Design review of the part built by this model. Coordinates are the model's own, in mm. Face numbers are marked on the shaded views. A direction names the side the tool comes from. Give positions to 0.01 mm unless a question says otherwise; leave off trailing zeros. Order: outer loops, then holes, each group sorted by start corner. A loop starts at its lowest first (then second) coordinate and runs counter-clockwise, first axis right, second up.
```python
from build123d import *

# Parameters (mm, degrees)
SKETCH1_R           = 14
BOSS_EXTRUDE1_DEPTH = 25
SKETCH3_R           = 4.5
BOSS_EXTRUDE2_DEPTH = 1
SKETCH4_R           = 1
CUT_EXTRUDE1_DEPTH  = 4
SKETCH5_R           = 1.5
CUT_EXTRUDE2_DEPTH  = 4


with BuildPart() as part:
    # Sketch1 → Boss-Extrude1 (new body)
    with BuildSketch(Plane(origin=(0, 0, 0), x_dir=(1, 0, 0), z_dir=(0, 1, 0))):
        with Locations(Location((0, 0, 0), (0, 0, 270))):
            Circle(SKETCH1_R)
    extrude(amount=BOSS_EXTRUDE1_DEPTH)

    # Sketch3 → Boss-Extrude2 (add)
    with BuildSketch(Plane(origin=(0, 25, 0), x_dir=(1, 0, 0), z_dir=(0, 1, 0))):
        with Locations(Location((0, 0, 0), (0, 0, 270))):
            Circle(SKETCH3_R)
    extrude(amount=BOSS_EXTRUDE2_DEPTH)

    # Sketch4 → Cut-Extrude1 (cut)
    with BuildSketch(Plane(origin=(0, 25, 0), x_dir=(1, 0, 0), z_dir=(0, 1, 0))):
        with Locations(Location((0, 5.773502692, 0), (0, 0, 270))):
            Circle(SKETCH4_R)
        with Locations(Location((5, -2.886751346, 0), (0, 0, 270))):
            Circle(SKETCH4_R)
        with Locations(Location((-5, -2.886751346, 0), (0, 0, 270))):
            Circle(SKETCH4_R)
    extrude(amount=-CUT_EXTRUDE1_DEPTH, mode=Mode.SUBTRACT)

    # Sketch5 → Cut-Extrude2 (cut)
    with BuildSketch(Plane.XZ):
        with Locations(Location((9.5, 0, 0), (0, 0, 270))):
            Circle(SKETCH5_R)
        with Locations(Location((-9.5, 0, 0), (0, 0, 270))):
            Circle(SKETCH5_R)
        with Locations(Location((0, -8, 0), (0, 0, 270))):
            Circle(SKETCH5_R)
        with Locations(Location((0, 8, 0), (0, 0, 270))):
            Circle(SKETCH5_R)
    extrude(amount=-CUT_EXTRUDE2_DEPTH, mode=Mode.SUBTRACT)


solid = part.part
```
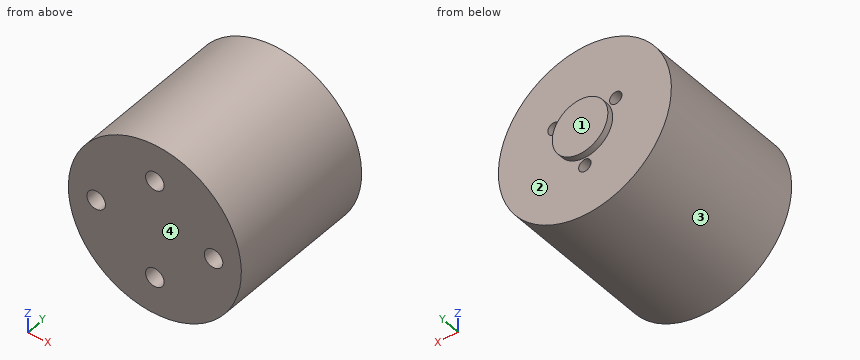
1. Take a section at D-D (y = 20). State the section outline as (x, z) points.
Recorded:
outline: circle Ø28 at (0, 0)
2. Draft analysis for pull direction Z (two halves, no side actions). For the marked faces 3 and 4, state which applies: pulls with the +Z half, pulls with the -Z half, needs draft (parallel to the pull), parting line crosses it, or undercut.
Recorded:
face 3: parting line crosses it
face 4: needs draft
3. Machinability: for the marked faces 1 and 2, which of the approach directions +Z, -Z, +X, -X, +Y, -Y give a long, thin tool a straight path to every point of the face, cutting with its end or side? Answer none if there is none.
Recorded:
face 1: +Z, -Z, +X, -X, +Y
face 2: +Y
4. For pin 1 (6 mm diameter, centred on x = 9, z = 9, fed in from +Y); pin 2 (0.9 mm diameter, centred on x = -0.5, z = -8.5, fed in from -Y); pin 3 (2 mm diameter, centred on y = 19, z = -5.5, fed in from -X), all flat-tipped, find the tip position at first contact; note any pin that passes through.
Recorded:
pin 1: stops at y = 25
pin 2: stops at y = 4
pin 3: stops at x = -13.26
5. Take a section at B-B (z = 0). State the section outline as (x, y) points, then the cut area to 3 significant figures.
Recorded:
outline: (-14, 0) - (-11, 0) - (-11, 4) - (-8, 4) - (-8, 0) - (8, 0) - (8, 4) - (11, 4) - (11, 0) - (14, 0) - (14, 25) - (4.5, 25) - (4.5, 26) - (-4.5, 26) - (-4.5, 25) - (-14, 25) - close
area: 685 mm2
6. For line 1 along X through (y, z) = (2.35, 0); line 2 along Y through (x, z) = (-5.75, -12.25); line 3 along X through (y, z) = (21.75, -5), list the stretches that pass through material, from the lowest coordinate up.
Recorded:
line 1: x = -14 to -11, -8 to 8, 11 to 14
line 2: y = 0 to 25
line 3: x = -13.08 to -0.63, 0.63 to 13.08
7. Take a section at C-C (y = 24). State the section outline as (x, z) points, then the cut area to 3 significant figures.
Recorded:
outline: circle Ø28 at (0, 0); hole circle Ø2 at (-5, 2.89); hole circle Ø2 at (0, -5.77); hole circle Ø2 at (5, 2.89)
area: 606 mm2
8. Take a section at A-A (x = 0). State the section outline as (y, z) points, then the cut area to 3 significant figures.
Recorded:
outline: (0, -14) - (25, -14) - (25, -6.77) - (21, -6.77) - (21, -4.77) - (25, -4.77) - (25, -4.5) - (26, -4.5) - (26, 4.5) - (25, 4.5) - (25, 14) - (0, 14) - (0, 9.5) - (4, 9.5) - (4, 6.5) - (0, 6.5) - (0, -6.5) - (4, -6.5) - (4, -9.5) - (0, -9.5) - close
area: 677 mm2
